Design review of the part built by this model. Coordinates are the model's own, in mm. Face numbers are marked on the shaded views. A direction names the side the tool comes from. Round coordinates to 2 decimals unless told otherwise and drop trailing zeros. Write each loop counter-clockwise with the first axis right and the second up, starting at its lowest first coordinate (ties: lowest second). Pieces come first, ordered by that corner, then holes. Notation, with made-up numbers: (52, 67) -> (65, 67) arc R24 cw to (65, 104) -> close; hole circle Ø11 at (-24.5, 7). An arc over 180 degrees is marked (long way). Write item = value, one per line. Start each with the question number.
Item 1: Add section D-D, the plane y = -23. State the section outline as (x, z) points.
Item 2: Add section C-C, the plane z = -6. State the section outline as (x, y) points.
Item 3: Machinability: for the marked faces 4, 5 and 6, which of the approach directions +Z, -Z, +X, -X, +Y, -Y give a long, thin tool a straight path to every point of the face, cutting with its end or side? Answer none if there is none.
Item 4: Add section B-B, the plane x = -19.5. State the section outline as (y, z) points, then the cut area to 3 significant figures.
Item 5: Mouldability with a two-part tool opening along X and no side actions: class the marked faces 1, 2 and 3 as released by +X, released by -X, zero draft, split by the parting line, or undercut.
Item 6: To check wall thickness, follow L1, parallel to X at y = -32, z = -11; L2, parallel to Z at x = 13, y = -23; L3, parallel to X at y = -26, z = 6. State the ranges of each line that lie inside material, in increasing order.
Item 7: For pin 1 Ø12.5 at (x, z) = (4, -4) entering from -Y; pin 2 Ø1 at (x, y) = (18, -10.5) entering from +Z; pin 3 Ø20.5 at (x, z) = (-28, 17.5) entering from +Y, all flat-tipped, find the tip position at first contact; note any pin that passes through.
Item 8: Add section A-A, the plane y = -34. State the section outline as (x, z) points.
from build123d import *

# Parameters (mm, degrees)
F0_W     = 25.4
F0_H     = 25.4
F1_DEPTH = 25.4
F2_DEPTH = 50.8
F3_W     = 25.4
F3_H     = 25.4
F4_DEPTH = 25.4


with BuildPart() as f1:
    # F0 (on Front) → F1 (new body)
    with BuildSketch(Plane.XZ):
        with Locations((-1.210593, -7.368315)):
            Rectangle(F0_W, F0_H)
    extrude(amount=F1_DEPTH)

    # F0 (on Front) → F2 (join)
    with BuildSketch(Plane.XZ):
        with Locations((-26.610593, -7.368315)):
            Rectangle(F0_W, F0_H)
        with Locations((24.189407, -7.368315)):
            Rectangle(F0_W, F0_H)
    extrude(amount=F2_DEPTH)

    # F3 (on face) → F4 (join)
    with BuildSketch(Plane.XY.offset(5.331685)):
        with Locations((-26.610593, -38.1)):
            Rectangle(F3_W, F3_H)
    extrude(amount=F4_DEPTH)


solid = f1.part
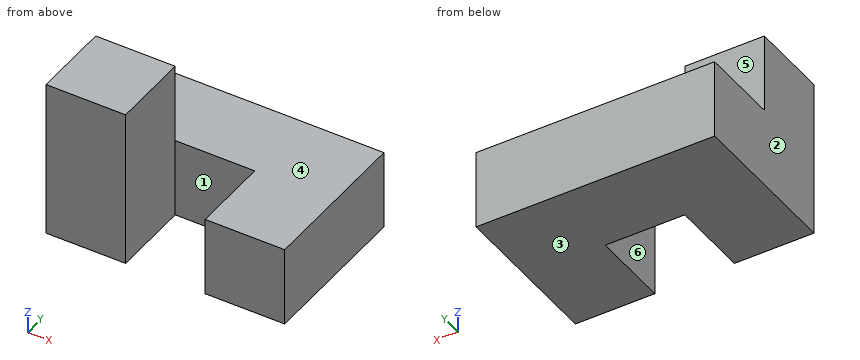
Result set:
q1.outline = (-39.31, -20.07) -> (36.89, -20.07) -> (36.89, 5.33) -> (-39.31, 5.33) -> close
q2.outline = (-39.31, -50.8) -> (-13.91, -50.8) -> (-13.91, -25.4) -> (11.49, -25.4) -> (11.49, -50.8) -> (36.89, -50.8) -> (36.89, 0) -> (-39.31, 0) -> close
q3.face_4 = +Z, +X, +Y
q3.face_5 = +Z, +X, -X, +Y
q3.face_6 = +Z, -Z, -Y
q4.outline = (-50.8, -20.07) -> (0, -20.07) -> (0, 5.33) -> (-25.4, 5.33) -> (-25.4, 30.73) -> (-50.8, 30.73) -> close
q4.area = 1,940 mm²
q5.face_1 = undercut
q5.face_2 = released by -X
q5.face_3 = zero draft
q6.L1 = -39.31 to -13.91, 11.49 to 36.89
q6.L2 = -20.07 to 5.33
q6.L3 = -39.31 to -13.91
q7.pin_1 = -25.4
q7.pin_2 = 5.33
q7.pin_3 = -25.4
q8.outline = (-39.31, -20.07) -> (-13.91, -20.07) -> (-13.91, 30.73) -> (-39.31, 30.73) -> close; (11.49, -20.07) -> (36.89, -20.07) -> (36.89, 5.33) -> (11.49, 5.33) -> close
